Geometry check sheet. Reference: the model listing, model coordinates, mm. Coordinates: 2 decimals unless noted, no trailing zeros. Loops run counter-clockwise (first coordinate to the right, second up) from the corner with the lowest first, then second, coordinate; pieces in that order, holes last.
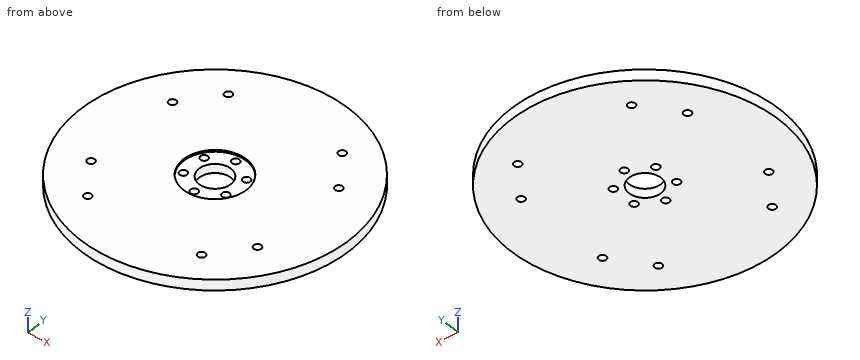
from build123d import *

# Parameters (mm, degrees)
SKETCH_1_R           = 40
EXTRUDE_1_DEPTH      = 2
SKETCH_2_R           = 34
CUT_EXTRUDE_1_DEPTH  = 0.5
SKETCH_3_R           = 17.5
CUT_EXTRUDE_4_DEPTH  = 1
SKETCH_5_R           = 2
CUT_EXTRUDE_5_DEPTH  = 1
SKETCH_6_R           = 8
CUT_EXTRUDE_6_DEPTH  = 10
SKETCH_7_R           = 2.1
CUT_EXTRUDE_7_DEPTH  = 10
SKETCH_8_R           = 70
SKETCH_8_R_2         = 40
EXTRUDE_2_DEPTH      = 2
EXTRUDE_3_DEPTH      = 2
SKETCH_11_R          = 75
SKETCH_11_R_2        = 2.1
SKETCH_11_R_3        = 8
EXTRUDE_4_DEPTH      = 2
SKETCH_13_W          = 95.696329608
SKETCH_13_H          = 36
SKETCH_13_W_2        = 36
SKETCH_13_H_2        = 100.137159233
SKETCH_13_H_3        = 96.241749767
CUT_EXTRUDE_10_DEPTH = 198
SKETCH_11_3_R        = 75
SKETCH_11_3_R_2      = 2.1
SKETCH_11_3_R_3      = 8
EXTRUDE_5_DEPTH      = 2
SKETCH_17_R          = 1.65
CUT_EXTRUDE_12_DEPTH = 280
SKETCH_18_R          = 234.864992374
SKETCH_18_R_2        = 75
SKETCH_18_R_3        = 1.65
CUT_EXTRUDE_13_DEPTH = 222
SKETCH_20_R          = 8.888358942
CUT_EXTRUDE_15_DEPTH = 17
SKETCH_28_R          = 17.5
CUT_EXTRUDE_16_DEPTH = 1
SKETCH_34_R          = 17.6
CUT_EXTRUDE_22_DEPTH = 1
SKETCH_30_R          = 2.1
CUT_EXTRUDE_27_DEPTH = 10
SKETCH_33_R          = 2.1
CUT_EXTRUDE_28_DEPTH = 10
EXTRUDE_START        = 4
SKETCH_40_R          = 75
SKETCH_40_R_2        = 8.888358942
SKETCH_40_R_3        = 2.1
EXTRUDE_6_DEPTH      = 4


with BuildPart() as part:
    # Sketch 1 → Extrude 1 (new body)
    with BuildSketch(Plane.XY):
        Circle(SKETCH_1_R)
    extrude(amount=EXTRUDE_1_DEPTH)

    # Sketch 2 → Cut-Extrude 1 (cut)
    with BuildSketch(Plane.XY.offset(2)):
        Circle(SKETCH_2_R)
    extrude(amount=-CUT_EXTRUDE_1_DEPTH, mode=Mode.SUBTRACT)

    # Sketch 3 → Cut-Extrude 4 (cut)
    with BuildSketch(Plane.XY.offset(1.5)):
        Circle(SKETCH_3_R)
    extrude(amount=-CUT_EXTRUDE_4_DEPTH, mode=Mode.SUBTRACT)

    # Sketch 5 → Cut-Extrude 5 (cut)
    with BuildSketch(Plane.XY.offset(0.5)):
        with Locations((0, 14)):
            Circle(SKETCH_5_R)
        with Locations((12.124355653, 7)):
            Circle(SKETCH_5_R)
        with Locations((12.124355653, -7)):
            Circle(SKETCH_5_R)
        with Locations((0, -14)):
            Circle(SKETCH_5_R)
        with Locations((-12.124355653, -7)):
            Circle(SKETCH_5_R)
        with Locations((-12.124355653, 7)):
            Circle(SKETCH_5_R)
    extrude(amount=-CUT_EXTRUDE_5_DEPTH, mode=Mode.SUBTRACT)

    # Sketch 6 → Cut-Extrude 6 (cut)
    with BuildSketch(Plane(origin=(0, 0, 0), x_dir=(-1, 0, 0), z_dir=(0, 0, -1))):
        Circle(SKETCH_6_R)
    extrude(amount=-CUT_EXTRUDE_6_DEPTH, mode=Mode.SUBTRACT)

    # Sketch 7 → Cut-Extrude 7 (cut)
    with BuildSketch(Plane(origin=(0, 0, 0), x_dir=(-1, 0, 0), z_dir=(0, 0, -1))):
        with Locations((0, 14)):
            Circle(SKETCH_7_R)
        with Locations((12.124355653, 7)):
            Circle(SKETCH_7_R)
        with Locations((12.124355653, -7)):
            Circle(SKETCH_7_R)
        with Locations((0, -14)):
            Circle(SKETCH_7_R)
        with Locations((-12.124355653, -7)):
            Circle(SKETCH_7_R)
        with Locations((-12.124355653, 7)):
            Circle(SKETCH_7_R)
    extrude(amount=-CUT_EXTRUDE_7_DEPTH, mode=Mode.SUBTRACT)

    # Sketch 8 → Extrude 2 (add)
    with BuildSketch(Plane(origin=(0, 0, 0), x_dir=(-1, 0, 0), z_dir=(0, 0, -1))):
        Circle(SKETCH_8_R)
        Circle(SKETCH_8_R_2, mode=Mode.SUBTRACT)
    extrude(amount=-EXTRUDE_2_DEPTH)

    # Sketch 9 → Extrude 3 (add)
    with BuildSketch(Plane(origin=(0, 0, 0), x_dir=(-1, 0, 0), z_dir=(0, 0, -1))):
        with BuildLine():
            ThreePointArc((-36.858328143, 59.510197836), (-0.940414163, 69.993682724), (35.246189577, 60.478972547))
            Line((35.246189577, 60.478972547), (35.246189577, 159.510197836))
            Line((35.246189577, 159.510197836), (-36.858328143, 159.510197836))
            Line((-36.858328143, 159.510197836), (-36.858328143, 59.510197836))
        make_face()
        with BuildLine():
            Line((160, 36.055512755), (60, 36.055512755))
            ThreePointArc((60, 36.055512755), (67.453687816, 18.708286934), (70, 0))
            ThreePointArc((70, 0), (67.453687816, -18.708286934), (60, -36.055512755))
            Line((60, -36.055512755), (160, -36.055512755))
            Line((160, -36.055512755), (160, 36.055512755))
        make_face()
        with BuildLine():
            ThreePointArc((35.246189577, -60.478972547), (-0.940414163, -69.993682724), (-36.858328143, -59.510197836))
            Line((-36.858328143, -59.510197836), (-36.858328143, -160.478972547))
            Line((-36.858328143, -160.478972547), (35.246189577, -160.478972547))
            Line((35.246189577, -160.478972547), (35.246189577, -60.478972547))
        make_face()
        with BuildLine():
            ThreePointArc((-60, -36.055512755), (-70, 0), (-60, 36.055512755))
            Line((-60, 36.055512755), (-160, 36.055512755))
            Line((-160, 36.055512755), (-160, -36.055512755))
            Line((-160, -36.055512755), (-60, -36.055512755))
        make_face()
    extrude(amount=-EXTRUDE_3_DEPTH)

    # Sketch 11 → Extrude 4 (add)
    with BuildSketch(Plane(origin=(0, 0, 0), x_dir=(-1, 0, 0), z_dir=(0, 0, -1))):
        Circle(SKETCH_11_R)
        with Locations((0, -14)):
            Circle(SKETCH_11_R_2, mode=Mode.SUBTRACT)
        with Locations((-12.124355653, -7)):
            Circle(SKETCH_11_R_2, mode=Mode.SUBTRACT)
        with Locations((-12.124355653, 7)):
            Circle(SKETCH_11_R_2, mode=Mode.SUBTRACT)
        Circle(SKETCH_11_R_3, mode=Mode.SUBTRACT)
        with Locations((12.124355653, -7)):
            Circle(SKETCH_11_R_2, mode=Mode.SUBTRACT)
        with Locations((12.124355653, 7)):
            Circle(SKETCH_11_R_2, mode=Mode.SUBTRACT)
        with Locations((0, 14)):
            Circle(SKETCH_11_R_2, mode=Mode.SUBTRACT)
    extrude(amount=-EXTRUDE_4_DEPTH)

    # Sketch 13 → Cut-Extrude 10 (cut)
    with BuildSketch(Plane(origin=(0, 0, 0), x_dir=(-1, 0, 0), z_dir=(0, 0, -1))):
        with Locations((-112.151835196, 0)):
            Rectangle(SKETCH_13_W, SKETCH_13_H)
        with Locations((0, 109.44161822)):
            Rectangle(SKETCH_13_W_2, SKETCH_13_H_2)
        Polygon((160, -18), (160, 18), (157.649128195, 18), (52.463986971, 18), (52.463986971, -18), align=None)
        with Locations((0, -112.358097664)):
            Rectangle(SKETCH_13_W_2, SKETCH_13_H_3)
    extrude(amount=-CUT_EXTRUDE_10_DEPTH, mode=Mode.SUBTRACT)

    # Sketch 11_3 → Extrude 5 (add)
    with BuildSketch(Plane(origin=(0, 0, 0), x_dir=(-1, 0, 0), z_dir=(0, 0, -1))):
        Circle(SKETCH_11_3_R)
        with Locations((0, -14)):
            Circle(SKETCH_11_3_R_2, mode=Mode.SUBTRACT)
        with Locations((-12.124355653, -7)):
            Circle(SKETCH_11_3_R_2, mode=Mode.SUBTRACT)
        with Locations((-12.124355653, 7)):
            Circle(SKETCH_11_3_R_2, mode=Mode.SUBTRACT)
        Circle(SKETCH_11_3_R_3, mode=Mode.SUBTRACT)
        with Locations((12.124355653, -7)):
            Circle(SKETCH_11_3_R_2, mode=Mode.SUBTRACT)
        with Locations((12.124355653, 7)):
            Circle(SKETCH_11_3_R_2, mode=Mode.SUBTRACT)
        with Locations((0, 14)):
            Circle(SKETCH_11_3_R_2, mode=Mode.SUBTRACT)
    extrude(amount=-EXTRUDE_5_DEPTH)

    # Sketch 17 → Cut-Extrude 12 (cut)
    with BuildSketch(Plane(origin=(0, 0, 0), x_dir=(-1, 0, 0), z_dir=(0, 0, -1))):
        with Locations((-27.027756377, 157.6)):
            Circle(SKETCH_17_R)
        with Locations((-27.027756377, 132.6)):
            Circle(SKETCH_17_R)
        with Locations((27.027756377, 132.6)):
            Circle(SKETCH_17_R)
        with Locations((132.6, 27.027756377)):
            Circle(SKETCH_17_R)
        with Locations((-27.027756377, -157.6)):
            Circle(SKETCH_17_R)
        with Locations((-157.6, 27.027756377)):
            Circle(SKETCH_17_R)
        with Locations((-132.6, 27.027756377)):
            Circle(SKETCH_17_R)
        with Locations((-157.6, -27.027756377)):
            Circle(SKETCH_17_R)
        with Locations((-132.6, -27.027756377)):
            Circle(SKETCH_17_R)
        with Locations((27.027756377, 157.6)):
            Circle(SKETCH_17_R)
        with Locations((157.6, 27.027756377)):
            Circle(SKETCH_17_R)
        with Locations((-27.027756377, -132.6)):
            Circle(SKETCH_17_R)
        with Locations((27.027756377, -132.6)):
            Circle(SKETCH_17_R)
        with Locations((27.027756377, -157.6)):
            Circle(SKETCH_17_R)
    extrude(amount=-CUT_EXTRUDE_12_DEPTH, mode=Mode.SUBTRACT)

    # Sketch 18 → Cut-Extrude 13 (cut)
    with BuildSketch(Plane(origin=(0, 0, 0), x_dir=(-1, 0, 0), z_dir=(0, 0, -1))):
        Circle(SKETCH_18_R)
        Circle(SKETCH_18_R_2, mode=Mode.SUBTRACT)
        with Locations((157.6, 27.027756377)):
            Circle(SKETCH_18_R_3, mode=Mode.SUBTRACT)
    extrude(amount=-CUT_EXTRUDE_13_DEPTH, mode=Mode.SUBTRACT)

    # Sketch 20 → Cut-Extrude 15 (cut)
    with BuildSketch(Plane(origin=(0, 0, 0), x_dir=(-1, 0, 0), z_dir=(0, 0, -1))):
        Circle(SKETCH_20_R)
    extrude(amount=-CUT_EXTRUDE_15_DEPTH, mode=Mode.SUBTRACT)

    # Sketch 28 → Cut-Extrude 16 (cut)
    with BuildSketch(Plane.XY.offset(2)):
        Circle(SKETCH_28_R)
    extrude(amount=-CUT_EXTRUDE_16_DEPTH, mode=Mode.SUBTRACT)

    # Sketch 34 → Cut-Extrude 22 (cut)
    with BuildSketch(Plane.XY.offset(2)):
        Circle(SKETCH_34_R)
    extrude(amount=-CUT_EXTRUDE_22_DEPTH, mode=Mode.SUBTRACT)

    # Sketch 30 → Cut-Extrude 27 (cut)
    with BuildSketch(Plane(origin=(0, 0, 0), x_dir=(-1, 0, 0), z_dir=(0, 0, -1))):
        with Locations((-32.5, -47.5)):
            Circle(SKETCH_30_R)
        with Locations((32.5, -47.5)):
            Circle(SKETCH_30_R)
        with Locations((-32.5, 47.5)):
            Circle(SKETCH_30_R)
        with Locations((32.5, 47.5)):
            Circle(SKETCH_30_R)
    extrude(amount=-CUT_EXTRUDE_27_DEPTH, mode=Mode.SUBTRACT)

    # Sketch 33 → Cut-Extrude 28 (cut)
    with BuildSketch(Plane(origin=(0, 0, 0), x_dir=(-1, 0, 0), z_dir=(0, 0, -1))):
        with Locations((-47.5, 27.5)):
            Circle(SKETCH_33_R)
        with Locations((-47.5, -27.5)):
            Circle(SKETCH_33_R)
        with Locations((47.5, 27.5)):
            Circle(SKETCH_33_R)
        with Locations((47.5, -27.5)):
            Circle(SKETCH_33_R)
    extrude(amount=-CUT_EXTRUDE_28_DEPTH, mode=Mode.SUBTRACT)

    # Sketch 40 → Extrude 6 (add)
    with BuildSketch(Plane(origin=(0, 0, 0), x_dir=(-1, 0, 0), z_dir=(0, 0, -1)).offset(EXTRUDE_START)):
        Circle(SKETCH_40_R)
        Circle(SKETCH_40_R_2, mode=Mode.SUBTRACT)
        with Locations((-12.124355653, 7)):
            Circle(SKETCH_40_R_3, mode=Mode.SUBTRACT)
        with Locations((-12.124355653, -7)):
            Circle(SKETCH_40_R_3, mode=Mode.SUBTRACT)
        with Locations((0, -14)):
            Circle(SKETCH_40_R_3, mode=Mode.SUBTRACT)
        with Locations((12.124355653, -7)):
            Circle(SKETCH_40_R_3, mode=Mode.SUBTRACT)
        with Locations((12.124355653, 7)):
            Circle(SKETCH_40_R_3, mode=Mode.SUBTRACT)
        with Locations((0, 14)):
            Circle(SKETCH_40_R_3, mode=Mode.SUBTRACT)
        with Locations((32.5, 47.5)):
            Circle(SKETCH_40_R_3, mode=Mode.SUBTRACT)
        with Locations((47.5, 27.5)):
            Circle(SKETCH_40_R_3, mode=Mode.SUBTRACT)
        with Locations((47.5, -27.5)):
            Circle(SKETCH_40_R_3, mode=Mode.SUBTRACT)
        with Locations((32.5, -47.5)):
            Circle(SKETCH_40_R_3, mode=Mode.SUBTRACT)
        with Locations((-32.5, -47.5)):
            Circle(SKETCH_40_R_3, mode=Mode.SUBTRACT)
        with Locations((-47.5, -27.5)):
            Circle(SKETCH_40_R_3, mode=Mode.SUBTRACT)
        with Locations((-47.5, 27.5)):
            Circle(SKETCH_40_R_3, mode=Mode.SUBTRACT)
        with Locations((-32.5, 47.5)):
            Circle(SKETCH_40_R_3, mode=Mode.SUBTRACT)
    extrude(amount=-EXTRUDE_6_DEPTH)


solid = part.part
1) Material ranges on probe 1 along Y at (x, z) = (0, -0.1); probe 2 along Y at (x, z) = (0.5, 0.45); probe 3 along X at (y, z) = (16.5, -2.65), recorded low to high.
Data:
probe 1: y = -75 to -16.1, -11.9 to -8.89, 8.89 to 11.9, 16.1 to 75
probe 2: y = -75 to -16.04, -11.96 to -8.87, 8.87 to 11.96, 16.04 to 75
probe 3: x = -73.16 to 73.16
2) Section check D-D on y = 27.5. Record the cut outline in (x, z).
Data:
outline: (-69.78, -4) - (-49.6, -4) - (-49.6, 2) - (-69.78, 2) - close; (-45.4, -4) - (45.4, -4) - (45.4, 2) - (-45.4, 2) - close; (49.6, -4) - (69.78, -4) - (69.78, 2) - (49.6, 2) - close
3) Section check C-C on y = 7. Record the cut outline in (x, z), and give its area (3 significant figures).
Data:
outline: (-74.67, -4) - (-14.22, -4) - (-14.22, 1) - (-16.15, 1) - (-16.15, 2) - (-74.67, 2) - close; (-10.02, -4) - (-5.48, -4) - (-5.48, 1) - (-10.02, 1) - close; (5.48, -4) - (10.02, -4) - (10.02, 1) - (5.48, 1) - close; (14.22, -4) - (74.67, -4) - (74.67, 2) - (16.15, 2) - (16.15, 1) - (14.22, 1) - close
area: 767 mm2
4) Depth check by flat-ended pin: pin 1 (4 mm diameter, centred on x = -32.5, y = -47.5, fed in from +Z); pin 2 (5 mm diameter, centred on x = 0, y = 14, fed in from -Z); pin 3 (5 mm diameter, centred on x = 12.12, y = 7, fed in from +Z). Enter the tip coordinate at first touch or a pass-through.
Data:
pin 1: passes through
pin 2: stops at z = -4
pin 3: stops at z = 1
5) Section check A-A on z = -1. Count the separate pieces of the cut face and the enclosed holes in it, and give its area (3 significant figures).
Data:
separate pieces: 1
enclosed holes: 15
area: 17,200 mm2
6) Section check B-B on x = 32.5. Record the cut outline in (y, z), and give its area (3 significant figures).
Data:
outline: (-67.59, -4) - (-49.6, -4) - (-49.6, 2) - (-67.59, 2) - close; (-45.4, -4) - (45.4, -4) - (45.4, 2) - (-45.4, 2) - close; (49.6, -4) - (67.59, -4) - (67.59, 2) - (49.6, 2) - close
area: 761 mm2
